```python
from build123d import *

# Parameters (mm, degrees)
BOSS_EXTRUDE1_DEPTH = 15
SKETCH2_R           = 5.25
CUT_EXTRUDE1_DEPTH  = 7
SKETCH3_R           = 3.25
CUT_EXTRUDE2_DEPTH  = 20


with BuildPart() as part:
    # Sketch1 → Boss-Extrude1 (new body)
    with BuildSketch(Plane(origin=(0, 0, 0), x_dir=(1, 0, 0), z_dir=(0, 1, 0))):
        with BuildLine():
            Line((57.5, 15), (-57.5, 15))
            Line((-57.5, 15), (-57.5, 1.25))
            Line((-57.5, 1.25), (-45.421567416, 1.25))
            ThreePointArc((-45.421567416, 1.25), (-34.873770875, 9.980372592), (-25.5, 0))
            ThreePointArc((-25.5, 0), (-34.873770875, -9.980372592), (-45.421567416, -1.25))
            Line((-45.421567416, -1.25), (-57.5, -1.25))
            Line((-57.5, -1.25), (-57.5, -15))
            Line((-57.5, -15), (57.5, -15))
            Line((57.5, -15), (57.5, -1.25))
            Line((57.5, -1.25), (45.421567416, -1.25))
            ThreePointArc((45.421567416, -1.25), (25.5, 0), (45.421567416, 1.25))
            Line((45.421567416, 1.25), (57.5, 1.25))
            Line((57.5, 1.25), (57.5, 15))
        make_face()
    extrude(amount=BOSS_EXTRUDE1_DEPTH)

    # Sketch2 → Cut-Extrude1 (cut)
    with BuildSketch(Plane(origin=(0, 0, -15), x_dir=(-1, 0, 0), z_dir=(0, 0, -1))):
        with Locations((-50.5, 7.5)):
            Circle(SKETCH2_R)
        with Locations((50.5, 7.5)):
            Circle(SKETCH2_R)
    extrude(amount=-CUT_EXTRUDE1_DEPTH, mode=Mode.SUBTRACT)

    # Sketch3 → Cut-Extrude2 (cut)
    with BuildSketch(Plane(origin=(0, 0, -8), x_dir=(-1, 0, 0), z_dir=(0, 0, -1))):
        with Locations((-50.5, 7.5)):
            Circle(SKETCH3_R)
        with Locations((50.5, 7.5)):
            Circle(SKETCH3_R)
    extrude(amount=-CUT_EXTRUDE2_DEPTH, mode=Mode.SUBTRACT)


solid = part.part
```
Check sheet for the modelled part. Datum: model origin and axes. Units: mm. A direction names the side the tool comes from. Round coordinates to 2 decimals unless told otherwise and drop trailing zeros. Order: outer loops, then holes, each group sorted by start corner. A loop starts at its lowest first (then second) coordinate and runs counter-clockwise, first axis right, second up.
1) Section check B-B (x = -50.5). Record the boundary of the cut face in (y, z), and give its area (3 significant figures).
2) Section check C-C (x = -35.5). Record the boundary of the cut face in (y, z).
3) Tool access check on faces 4 (the cylindrical face through (-53.6, 8.48, -4.67)), 5 (the flat face through (54, 7, -1.25)), 6 (the flat face through (-54, 7, 1.25)). Record the directions out of +Z, -Z, +X, -X, +Y, -Y that give a thin tool (end or side, any length) a straight path to the whole face; none if there is none.
4) Mould release check, pull along Z, two halves, no side actions. Record for faces 1 (the flat face through (54, 7, 1.25)), 2 (the flat face through (1, 7, -15)), 3 (the flat face through (57.5, 7, -8)): +Z half, -Z half, draft (parallel to the pull), parting line (faces both ways), or undercut.
5) Section check D-D (z = 2.25). Record the boundary of the cut face in (x, y), and give its area (3 significant figures).
6) Go/stop test with flat-tipped pins: pin 1 Ø3 at (x, y) = (-50.5, 5) entering from -Z; pin 2 Ø6 at (x, y) = (-50.5, 7.5) entering from -Z; pin 3 Ø18 at (x, z) = (35.5, 0) entering from -Y. Record where each tip stops, or that it passes through.
7) Scan lines: line 1 (Y direction, x = -50.5, z = -12.25); line 2 (Y direction, x = -50.5, z = -4.25); line 3 (X direction, y = 4.5, z = -6.5). Record each from-to range of solid material in increasing order.
8) Section check A-A (z = 7.5). Record the boundary of the cut face in (x, y).
Result:
1. outline: (0, -15) - (2.25, -15) - (2.25, -8) - (4.25, -8) - (4.25, -1.25) - (0, -1.25) - close; (0, 1.25) - (4.25, 1.25) - (4.25, 12) - (10.75, 12) - (10.75, 1.25) - (15, 1.25) - (15, 15) - (0, 15) - close; (10.75, -8) - (12.75, -8) - (12.75, -15) - (15, -15) - (15, -1.25) - (10.75, -1.25) - close
1. area: 225 mm2
2. outline: (0, -15) - (15, -15) - (15, -10) - (0, -10) - close; (0, 10) - (15, 10) - (15, 15) - (0, 15) - close
3. face 4: -Z
3. face 5: +X, +Y, -Y
3. face 6: -X, +Y, -Y
4. face 1: undercut
4. face 2: -Z half
4. face 3: draft
5. outline: (-57.5, 0) - (-45.24, 0) - (-45.24, 15) - (-57.5, 15) - close; (-25.76, 0) - (25.76, 0) - (25.76, 15) - (-25.76, 15) - close; (45.24, 0) - (57.5, 0) - (57.5, 15) - (45.24, 15) - close; hole circle Ø6.5 at (-50.5, 7.5); hole circle Ø6.5 at (50.5, 7.5)
5. area: 1,070 mm2
6. pin 1: stops at z = -8
6. pin 2: stops at z = 12
6. pin 3: passes through
7. line 1: y = 0 to 2.25, 12.75 to 15
7. line 2: y = 0 to 4.25, 10.75 to 15
7. line 3: x = -57.5 to -51.75, -49.25 to -43.1, -27.9 to 27.9, 43.1 to 49.25, 51.75 to 57.5
8. outline: (-57.5, 0) - (-42.11, 0) - (-42.11, 15) - (-57.5, 15) - close; (-28.89, 0) - (28.89, 0) - (28.89, 15) - (-28.89, 15) - close; (42.11, 0) - (57.5, 0) - (57.5, 15) - (42.11, 15) - close; hole circle Ø6.5 at (-50.5, 7.5); hole circle Ø6.5 at (50.5, 7.5)
